Part model, mm, in its own coordinate system. A direction names the side the tool comes from. Give positions to 0.01 mm unless a question says otherwise; leave off trailing zeros. Write each loop counter-clockwise with the first axis right and the second up, starting at its lowest first coordinate (ties: lowest second). Pieces come first, ordered by that corner, then holes.
from build123d import *

# Parameters (mm, degrees)
SKETCH1_W           = 20
SKETCH1_H           = 30
BOSS_EXTRUDE1_DEPTH = 5
SKETCH2_R           = 2.55
CUT_EXTRUDE1_DEPTH  = 19.708286934
SKETCH3_W           = 5
SKETCH3_H           = 30
BOSS_EXTRUDE2_DEPTH = 9
SKETCH4_R           = 8
CUT_EXTRUDE2_DEPTH  = 29.653097564
SKETCH5_R           = 1.25
CUT_EXTRUDE3_DEPTH  = 10
FILLET1_R           = 1


with BuildPart() as part:
    # Sketch1 → Boss-Extrude1 (new body)
    with BuildSketch(Plane(origin=(0, 0, 0), x_dir=(1, 0, 0), z_dir=(0, 1, 0))):
        Rectangle(SKETCH1_W, SKETCH1_H)
    extrude(amount=BOSS_EXTRUDE1_DEPTH)

    # Sketch2 → Cut-Extrude1 (cut, through all)
    with BuildSketch(Plane(origin=(0, 5, 0), x_dir=(1, 0, 0), z_dir=(0, 1, 0))):
        with Locations(Location((0, 10, 0), (0, 0, 270))):
            Circle(SKETCH2_R)
        with Locations(Location((0, -10, 0), (0, 0, 270))):
            Circle(SKETCH2_R)
    extrude(amount=-CUT_EXTRUDE1_DEPTH, mode=Mode.SUBTRACT)

    # Sketch3 → Boss-Extrude2 (add)
    with BuildSketch(Plane(origin=(0, 5, 0), x_dir=(1, 0, 0), z_dir=(0, 1, 0))):
        with Locations((-7.5, 0)):
            Rectangle(SKETCH3_W, SKETCH3_H)
    boss_extrude2 = extrude(amount=BOSS_EXTRUDE2_DEPTH)

    # Sketch4 → Cut-Extrude2 (cut, through all)
    with BuildSketch(Plane.ZY.offset(10)):
        with Locations((0, 14)):
            Circle(SKETCH4_R)
    cut_extrude2 = extrude(amount=-CUT_EXTRUDE2_DEPTH, mode=Mode.SUBTRACT)

    # Sketch5 → Cut-Extrude3 (cut)
    with BuildSketch(Plane(origin=(0, 14, 0), x_dir=(1, 0, 0), z_dir=(0, 1, 0))):
        with Locations(Location((-7.5, 11.5, 0), (0, 0, 270))):
            Circle(SKETCH5_R)
        with Locations(Location((-7.5, -11.5, 0), (0, 0, 270))):
            Circle(SKETCH5_R)
    cut_extrude3 = extrude(amount=-CUT_EXTRUDE3_DEPTH, mode=Mode.SUBTRACT)

    # Mirror1: Boss-Extrude2, Cut-Extrude2, Cut-Extrude3 across plane
    add(boss_extrude2.mirror(Plane(origin=(0, 0, 0), x_dir=(0, 0, 1), z_dir=(1, 0, 0))))
    add(cut_extrude2.mirror(Plane(origin=(0, 0, 0), x_dir=(0, 0, 1), z_dir=(1, 0, 0))), mode=Mode.SUBTRACT)
    add(cut_extrude3.mirror(Plane(origin=(0, 0, 0), x_dir=(0, 0, 1), z_dir=(1, 0, 0))), mode=Mode.SUBTRACT)

    # Fillet1
    fillet1_edges = [part.edges().sort_by_distance(p)[0] for p in [
        (-10, 7, -15),
        (10, 7, -15),
        (10, 7, 15),
        (-10, 7, 15),
        (-7.5, 14, -15),
        (7.5, 14, -15),
        (7.5, 14, 15),
        (-7.5, 14, 15),
    ]]
    fillet(fillet1_edges, radius=FILLET1_R)


solid = part.part
1) Drill centre lines: L1, parallel to X at y = 10.5, z = -11.5; L2, parallel to X at y = 6.5, z = 7; L3, parallel to Z at x = 7, y = 11. Where is each one in solid material? Low to high.
Check result:
L1: x = -10 to -8.75, -6.25 to -5, 5 to 6.25, 8.75 to 10
L2: x = -10 to -5, 5 to 10
L3: z = -15 to -12.65, -10.35 to -7.42, 7.42 to 10.35, 12.65 to 15
2) Saw through at D-D (x = -7.5). Write the cut outline in (y, z).
Check result:
outline: (0, -15) - (13, -15) arc R1 ccw to (14, -14) - (14, -12.75) - (4, -12.75) - (4, -10.25) - (14, -10.25) - (14, -8) arc R8 cw to (14, 8) - (14, 10.25) - (4, 10.25) - (4, 12.75) - (14, 12.75) - (14, 14) arc R1 ccw to (13, 15) - (0, 15) - close
3) Saw through at A-A (x = 0). Write the cut outline in (y, z).
Check result:
outline: (0, -15) - (5, -15) - (5, -12.55) - (0, -12.55) - close; (0, -7.45) - (5, -7.45) - (5, 7.45) - (0, 7.45) - close; (0, 12.55) - (5, 12.55) - (5, 15) - (0, 15) - close
4) Saw through at C-C (z = -8.5). Write the cut outline in (x, y), and give its area (3 significant figures).
Check result:
outline: (-10, 0) - (-2.06, 0) - (-2.06, 5) - (-5, 5) - (-5, 14) - (-10, 14) - close; (2.06, 0) - (10, 0) - (10, 14) - (5, 14) - (5, 5) - (2.06, 5) - close
area: 169 mm2
5) Mould opens along X. For faces 4 (the cylindrical face through (-9.699, 6.902, -14.715)), 5 (the cylindrical face through (7.465, 13.699, 14.715)), 6 (the cylindrical face through (8.26, 9.07, -12.49)), 7 (the cylindrical face through (9.715, 6.902, 14.699)) say: +X half, -X half, draft (parallel to the pull), parting line (faces both ways), or undercut.
Check result:
face 4: -X half
face 5: draft
face 6: undercut
face 7: +X half
6) Saw through at B-B (y = 7). Write the cut outline in (x, z).
Check result:
outline: (-10, -14) arc R1 ccw to (-9, -15) - (-5, -15) - (-5, -3.87) - (-10, -3.87) - close; (-10, 3.87) - (-5, 3.87) - (-5, 15) - (-9, 15) arc R1 ccw to (-10, 14) - close; (5, -15) - (9, -15) arc R1 ccw to (10, -14) - (10, -3.87) - (5, -3.87) - close; (5, 3.87) - (10, 3.87) - (10, 14) arc R1 ccw to (9, 15) - (5, 15) - close; hole circle Ø2.5 at (-7.5, -11.5); hole circle Ø2.5 at (-7.5, 11.5); hole circle Ø2.5 at (7.5, -11.5); hole circle Ø2.5 at (7.5, 11.5)
7) Flat gauge pins, fed straight in: P1, Ø3, axis at x = 7.5, z = -11.5, coming from the -Y side; P2, Ø4, axis at x = 0, z = -10, coming from the -Y side; P3, Ø8, axis at x = 0, z = 10, coming from the +Y side; P4, Ø1.2, axis at x = 7.5, z = 11.5, coming from the +Y side. Where does each tip first touch, or does it go through?
Check result:
P1: stops at y = 0
P2: passes through
P3: stops at y = 5
P4: stops at y = 4
8) 3-axis set-ups, long thin cutter, end or side, ignore diameter. For faces 1 (the flat face through (-7, 4, -12)), 2 (the flat face through (5, 5.4, 0.2)), 3 (the flat face through (8, 14, -10)): which of +Z, -Z, +X, -X, +Y, -Y reach the whole face in a straight line?
Check result:
face 1: +Y
face 2: +Z, -Z, +Y
face 3: +Z, -Z, +X, -X, +Y
